Geometry check sheet. Reference: the model listing, model coordinates, mm. Face numbers are marked on the shaded views. Round coordinates to 2 decimals unless told otherwise and drop trailing zeros. Loops run counter-clockwise (first coordinate to the right, second up) from the corner with the lowest first, then second, coordinate; pieces in that order, holes last.
```python
from build123d import *

# Parameters (mm, degrees)
CHAMFER_2_SIZE = 2


with BuildPart() as part:
    # Эскиз1 → Повернуть1 (revolve)
    with BuildSketch(Plane(origin=(0, 0, 0), x_dir=(0, 0, -1), z_dir=(1, 0, 0)), mode=Mode.PRIVATE) as revolve_1_sk:
        Polygon((8.85, 50), (-10, 50), (-10, 72.5), (0, 72.5), (0, 68), (93, 68), (93, 60), (83.15, 60), (83.15, 62), (79, 62), (79, 60), (30, 60), (30, 50), (27, 50), (27, 41), (22, 41), (22, 50), (12, 50), (12, 51.75), (8.85, 51.75), align=None)
    revolve(revolve_1_sk.sketch.rotate(Axis((0, 0, 0), (0, 0, -1)), 90), axis=Axis((0, 0, 0), (0, 0, -1)))

    # Фаска2
    chamfer_2_edges = [part.edges().sort_by_distance(p)[0] for p in [
        (-60, 0, -93),
        (-50, 0, 10),
        (-72.5, 0, 10),
    ]]
    chamfer(chamfer_2_edges, length=CHAMFER_2_SIZE)


solid = part.part
```
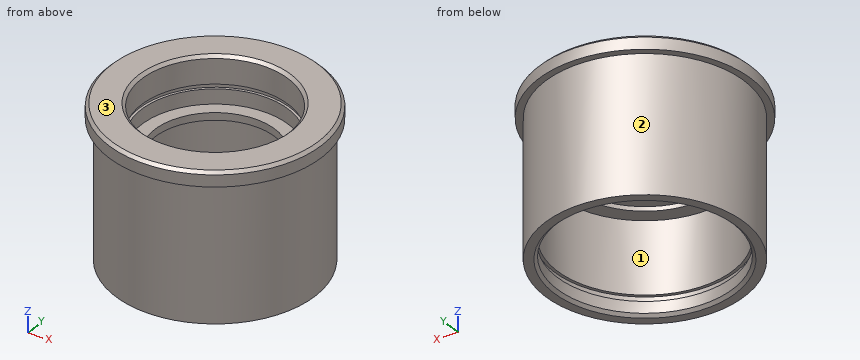
1) Scan lines: line 1 along Y through (x, z) = (0, -28); line 2 along Y through (x, z) = (-0.5, -33.5); line 3 along Z through (x, y) = (2, 47.5). Record each from-to range of solid material in increasing order.
Report:
line 1: y = -68 to -50, 50 to 68
line 2: y = -68 to -60, 60 to 68
line 3: z = -27 to -22
2) Gauge pin test, flat ends, axial feed: pin 1 (1.5 mm diameter, centred on y = -54.5, z = -52.5, fed in from +X); pin 2 (3 mm diameter, centred on y = 29.5, z = -37, fed in from -X); pin 3 (4 mm diameter, centred on x = 49.5, z = -22, fed in from +Y). Record the tip position at first contact, or that the pin passes through.
Report:
pin 1: stops at x = 41.65
pin 2: stops at x = -61.97
pin 3: stops at y = 48.66
3) Sectioned sample at B-B, the plane z = -50. Record the cut outline in (x, y), then the cut area to 3 significant figures.
Report:
outline: circle Ø136 at (0, 0); hole circle Ø120 at (0, 0)
area: 3,220 mm2
4) Mould release check, pull along X, two halves, no side actions. Record for the marked faces 1, 2 and 3: +X half, -X half, draft (parallel to the pull), parting line (faces both ways), or undercut.
Report:
face 1: undercut
face 2: parting line
face 3: draft
5) Sectioned sample at A-A, the plane z = -3. Record the cut outline in (x, y), then the cut area to 3 significant figures.
Report:
outline: circle Ø136 at (0, 0); hole circle Ø100 at (0, 0)
area: 6,670 mm2
